Geometry check sheet. Reference: the model listing, model coordinates, mm. A direction names the side the tool comes from. Give positions to 0.01 mm unless a question says otherwise; leave off trailing zeros. Write each loop counter-clockwise with the first axis right and the second up, starting at its lowest first coordinate (ties: lowest second). Pieces come first, ordered by that corner, then holes. Notation, with made-up numbers: (84.5, 36) - (119.5, 36) arc R17 ccw to (119.5, 44) - close; hole circle Ø5 at (35.25, -36). An arc over 180 degrees is marked (long way). Write item = value, one per line. Start each with the question number.
(1) Section check D-D, the plane x = 29.5. Enter the section's corners in (y, z), plus the area to 3 significant figures.
(2) Draft check along X on faces 1 (the cylindrical face through (17.23, 12.14, 1.48)), 2 (the cylindrical face through (14.8, 10.6, 1.5)), 3 (the flat face through (29, 15, 2)), 4 (the flat face through (34.521, 15.878, 1.986)). Enter one of: pulls with the +X half, pulls with the -X half, needs draft (parallel to the pull), parting line crosses it, or undercut.
(3) Section check A-A, the plane y = 13. Enter the section's corners in (x, z).
(4) Section check C-C, the plane x = 22. Enter the section's corners in (y, z), plus the area to 3 significant figures.
(5) Thickness scan on L1, parallel to X at y = 13, z = 1.6; L2, parallel to X at y = 13, z = 0.6; L3, parallel to X at y = 5, z = 2.1. Record the ranges inside material, lowest first.
(6) Depth check by flat-ended pin: pin 1 Ø4.5 at (x, y) = (9, 10) entering from -Z; pin 2 Ø3 at (x, y) = (4, 13) entering from +Z; pin 3 Ø3 at (x, y) = (17, 16) entering from -Z; pin 4 Ø3 at (x, y) = (3, 21) entering from -Z. Enter the tip coordinate at first touch or a pass-through.
(7) Access from +Z, -Z, +X, -X, +Y, -Y to the whole of each face (thin tool, end or side, straight path). Record for faces 5 (the cylindrical face through (3.64, 11.855, 0.961)), 6 (the cylindrical face through (7.5, 10.9, 0.5)).
(8) Section check B-B, the plane x = 12. Enter the section's corners in (y, z), plus the area to 3 significant figures.
Autodesk Inventor part; units mm, degrees
ref_plane "YZ Plane" through (0, 0, 0) normal (1, 0, 0) x (0, 1, 0)
ref_plane "XZ Plane" through (0, 0, 0) normal (0, 1, 0) x (-1, 0, 0)
ref_plane "XY Plane" through (0, 0, 0) normal (0, 0, 1) x (1, 0, 0)
sketch "Skizze1" plane through (0, 0, 0) normal (0, 0, 1) x (1, 0, 0)
  line L0 (-7.2, 0) -> (43.2, 0)
  line L1 (0, -4.6) -> (0, 27.6)
  line L2 (0, 23) -> (36, 23)
  line L3 (36, 23) -> (36, 0)
  line L4 (36, 0) -> (0, 0)
  line L5 (0, 0) -> (0, 23)
  point P0 (0, 0)
  dimension "d0" = 36
  dimension "d1" = 23
extrude "Extrusion1" add sketch "Skizze1" along normal blind 3
hole "Bohrung1" at (13, 13, 0) direction (0, 0, 1) diameter 6 end through all
sketch "Skizze3" plane through (0, 0, 3) normal (0, 0, 1) x (1, 0, 0)
  line L0 (19, 18) -> (7, 18)
  line L1 (7, 18) -> (7, 8)
  line L2 (19, 8) -> (19, 18)
  line L3 (7, 8) -> (19, 8)
  circle A0 centre (17, 16) radius 1.25
  circle A1 centre (9, 10) radius 1.25
  circle A2 centre (17.5, 13) radius 0.6105
  circle A3 centre (8.5, 13) radius 0.6105
  point P0 (8.5, 13)
  point P1 (17.5, 13)
hole "Bohrung2" at (8.5, 13, 3) at (17.5, 13, 3) direction (0, 0, -1) diameter 1.8 end through all
sketch "Skizze5" plane through (0, 0, 0) normal (0, 0, -1) x (-1, 0, 0)
  circle A0 centre (-17, 16) radius 1.25
  circle A1 centre (-9, 10) radius 1.25
  point P0 (-17, 16)
  point P1 (-9, 10)
hole "Bohrung3" at (17, 16, 0) at (9, 10, 0) direction (0, 0, 1) diameter 3.5 depth 1 tip angle 118
sketch "Skizze6" plane through (0, 23, 0) normal (0, 1, 0) x (1, 0, 0)
  line L0 (0, 0) -> (36, 0)
  line L1 (0, 0) -> (0, -3)
  line L2 (36, -3) -> (0, -3)
  line L3 (36, 0) -> (36, -3)
extrude "Extrusion2" add sketch "Skizze6" along normal blind 3
sketch "Skizze7" plane through (0, 0, 0) normal (0, 0, -1) x (-1, 0, 0)
  line L0 (-36, 26) -> (-36, 0)
  line L1 (-36, 0) -> (0, 0)
  line L2 (0, 0) -> (0, 26)
  line L3 (-36, 26) -> (0, 26)
  line L4 (-36, 25.9998) -> (0, 25.9998)
  line L5 (-6, 23) -> (-6, 3)
  line L6 (-26, 3) -> (-26, 23)
  line L7 (-36, 23) -> (0, 23)
  line L8 (0, 0) -> (-36, 0)
  line L9 (-6, 3) -> (-26, 3)
  line L10 (-6.5, 9) -> (-6.5, 17)
  arc A0 (-6.5, 17) -> (-8, 18.5) centre (-8, 17) ccw
  line L11 (-8, 18.5) -> (-10.0314, 18.5)
  line L12 (-15.9686, 18.5) -> (-18, 18.5)
  arc A1 (-18, 18.5) -> (-19.5, 17) centre (-18, 17) ccw
  line L13 (-19, 8) -> (-19, 18)
  line L14 (-16.2253, 8) -> (-19, 8)
  line L15 (-19.5, 17) -> (-19.5, 16)
  arc A2 (-19.5, 16) -> (-18, 7.5) centre (-18, 9) ccw
  arc A3 (-10.0314, 7.5) -> (-10.0314, 18.5) centre (-13, 13) ccw
  line L16 (-18, 7.5) -> (-15.9686, 7.5)
  line L17 (-10.0314, 7.5) -> (-8, 7.5)
  arc A4 (-8, 7.5) -> (-6.5, 9) centre (-8, 9) ccw
  line L18 (-6.5, 9) -> (-6.5, 17)
  line L19 (-3, 0) -> (-3, 25.9998)
  line L20 (-33, 25.9998) -> (-33, 0)
  line L21 (-33, 21) -> (-3, 21)
  line L22 (-3, 21) -> (-3, 5)
  line L23 (-3, 5) -> (-33, 5)
  line L24 (-33, 5) -> (-33, 21)
  line L25 (-36, 13) -> (0, 13)
  point P0 (-6, 23)
  dimension "d29" = 6
  dimension "d30" = 3
  dimension "d31" = 3
  dimension "d32" = 16
hole "Bohrung4" at (3, 21, 0) at (3, 5, 0) at (33, 21, 0) at (33, 5, 0) direction (0, 0, 1) diameter 2.4 end through all countersink diameter 4.5 countersink angle 90
sketch "Skizze9" plane through (0, 0, 3) normal (0, 0, 1) x (1, 0, 0)
  line L0 (0, 0) -> (0, 26)
  line L1 (36, 0) -> (36, 26)
  line L2 (3, 8) -> (2, 8)
  line L3 (2, 8) -> (2, 18)
  line L4 (2, 18) -> (3, 18)
  arc A0 (3, 18) -> (6, 21) centre (3, 21) ccw
  line L5 (6, 21) -> (6, 23)
  line L6 (6, 3) -> (6, 5)
  arc A1 (6, 5) -> (3, 8) centre (3, 5) ccw
  line L7 (0, 13) -> (36, 13)
  line L8 (22, 20.2065) -> (22, 3.5507)
  line L9 (6, 23) -> (30, 23)
  line L10 (30, 3) -> (30, 5)
  line L11 (6, 3) -> (30, 3)
  arc A2 (30, 21) -> (33, 18) centre (33, 21) ccw
  line L12 (34, 18) -> (33, 18)
  line L13 (34, 8) -> (34, 18)
  line L14 (33, 8) -> (34, 8)
  arc A3 (33, 8) -> (30, 5) centre (33, 5) ccw
  line L15 (30, 21) -> (30, 23)
  point P0 (22, 19)
  point P1 (22, 7)
  point P2 (4, 13)
  dimension "d41" = 22
  dimension "d42" = 14
  dimension "d43" = 12
  dimension "d44" = 4
hole "Bohrung5" at (22, 19, 3) at (22, 7, 3) at (4, 13, 3) direction (0, 0, -1) diameter 2.4 end through all countersink diameter 4.5 countersink angle 90
sketch "Skizze10" plane through (0, 0, 3) normal (0, 0, 1) x (1, 0, 0)
  circle A0 centre (22, 19) radius 2.25
  line L0 (36, 0) -> (36, 26)
  line L1 (0, 26) -> (36, 26)
  line L2 (36, 13) -> (19.5709, 13)
  line L3 (36, 11) -> (22, 11)
  line L4 (36, 15) -> (22, 15)
  line L5 (22, 15) -> (22, 11)
  line L6 (22, 19) -> (22, 15.7462)
  dimension "d52" = 4
extrude "Extrusion3" cut sketch "Skizze10" against normal blind 2 contours L3 L5 L2 L0 | L2 L5 L4 L0
sketch "Skizze11" plane through (0, 0, 3) normal (0, 0, 1) x (1, 0, 0)
  line L0 (22, 11) -> (22, 15)
  point P0 (22, 13)
hole "Bohrung6" at (22, 13, 3) direction (0, 0, -1) diameter 6 end through all
chamfer "Fase1" distance 3 angle 30 1 edges at (36, 11, 2) measured on face at (28.1574, 11, 2.3333)
chamfer "Fase2" distance 3 angle 30 1 edges at (36, 15, 2) measured on face at (32.0787, 15, 2.3333)
properties part number "13_1087_012"
Model answer:
q1.outline = (0, 0) - (26, 0) - (26, 3) - (15, 3) - (15, 1) - (11, 1) - (11, 3) - (0, 3) - close
q1.area = 70.0 mm²
q2.face_1 = undercut
q2.face_2 = undercut
q2.face_3 = needs draft
q2.face_4 = pulls with the +X half
q3.outline = (0, 0) - (2.8, 0) - (2.8, 1.95) - (1.75, 3) - (0, 3) - close; (5.2, 0) - (7.6, 0) - (7.6, 3) - (6.25, 3) - (5.2, 1.95) - close; (9.4, 0) - (10, 0) - (10, 3) - (9.4, 3) - close; (16, 0) - (16.6, 0) - (16.6, 3) - (16, 3) - close; (18.4, 0) - (19, 0) - (19, 3) - (18.4, 3) - close; (25, 0) - (36, 0) - (36, 1) - (25, 1) - close
q4.outline = (0, 0) - (5.8, 0) - (5.8, 1.95) - (4.75, 3) - (0, 3) - close; (8.2, 0) - (10, 0) - (10, 3) - (9.25, 3) - (8.2, 1.95) - close; (16, 0) - (17.8, 0) - (17.8, 1.95) - (16.75, 3) - (16, 3) - close; (20.2, 0) - (26, 0) - (26, 3) - (21.25, 3) - (20.2, 1.95) - close
q4.area = 43.4 mm²
q5.L1 = 0 to 2.8, 5.2 to 7.6, 9.4 to 10, 16 to 16.6, 18.4 to 19
q5.L2 = 0 to 2.8, 5.2 to 7.6, 9.4 to 10, 16 to 16.6, 18.4 to 19, 25 to 36
q5.L3 = 0 to 1.8, 4.2 to 31.8, 34.2 to 36
q6.pin_1 = 0
q6.pin_2 = 2.25
q6.pin_3 = 1.15
q6.pin_4 = 0.75
q7.face_5 = +Z, -Z
q7.face_6 = -Z
q8.outline = (0, 0) - (10.17, 0) - (10.17, 3) - (0, 3) - close; (15.83, 0) - (26, 0) - (26, 3) - (15.83, 3) - close
q8.area = 61.0 mm²
